Geometry: final body of the model. Coordinates: model frame, mm. A direction names the side the tool comes from. Coordinates: 2 decimals unless noted, no trailing zeros. Order: outer loops, then holes, each group sorted by start corner. A loop starts at its lowest first (then second) coordinate and runs counter-clockwise, first axis right, second up. Notation, with made-up numbers: (75.5, -27) - (94.5, -27) arc R23 ccw to (94.5, 7) - close; hole circle Ø2 at (70, 63.25). An arc over 180 degrees is marked (long way). Use a Markdown table: item, result. Add a question column.
Autodesk Inventor part; units mm, degrees
ref_plane "Work Plane1" through (0, 20, 0) normal (0, -1, 0) x (1, 0, 0)
ref_plane "YZ Plane" through (0, 0, 0) normal (1, 0, 0) x (0, 1, 0)
ref_plane "XZ Plane" through (0, 0, 0) normal (0, 1, 0) x (-1, 0, 0)
sketch "Sketch1" plane through (0, 0, 0) normal (0, 1, 0) x (-1, 0, 0)
  circle A0 centre (0, 0) radius 34.5
  dimension "d0" = 69
extrude "Extrusion1" add sketch "Sketch1" along normal blind 33.9
sketch "Sketch2" plane through (0, 33.9, 0) normal (0, 1, 0) x (1, 0, 0)
  circle A0 centre (0, 0) radius 34.5
  line L0 (-15, -15) -> (15, -15)
  line L1 (15, -15) -> (15, 15)
  line L2 (15, 15) -> (-15, 15)
  line L3 (-15, 15) -> (-15, -15)
  line L4 (-15, -15) -> (15, 15) construction
  line L5 (15, -15) -> (-15, 15) construction
  circle A1 centre (-15, 15) radius 1.5
  circle A2 centre (15, 15) radius 1.5
  circle A3 centre (-15, -15) radius 1.5
  circle A4 centre (15, -15) radius 1.5
  dimension "d3" = 30
  dimension "d4" = 30
  dimension "d5" = 3
  dimension "d6" = 3
  dimension "d7" = 3
  dimension "d8" = 3
hole "Hole1" at (-15, 33.9, 15) at (15, 33.9, 15) at (-15, 33.9, -15) at (15, 33.9, -15) direction (0, -1, 0) diameter 3 depth 10.4
sketch "Sketch3" plane through (0, 0, 0) normal (0, -1, 0) x (1, 0, 0)
  circle A0 centre (0, 0) radius 34.5
  circle A1 centre (0, 0) radius 6.35
  dimension "d16" = 12.7
extrude "Extrusion2" cut sketch "Sketch3" against normal blind 20 contours A1
ref_plane "Work Plane1" through (0, 20, 0) normal (0, -1, 0) x (1, 0, 0)
sketch "Sketch4" plane through (0, 20, 0) normal (0, -1, 0) x (1, 0, 0)
  circle A0 centre (0, 0) radius 6.35
  circle A1 centre (0, 0) radius 34.5
  circle A2 centre (0, 0) radius 34
  dimension "d20" = 68
extrude "Extrusion3" cut sketch "Sketch4" along normal mid plane 2 contours A1
sketch "Sketch5" plane through (0, 0, 0) normal (0, -1, 0) x (1, 0, 0)
  circle A0 centre (0, 0) radius 6.35
  circle A1 centre (0, 0) radius 34.5
  circle A2 centre (0, 0) radius 12.5
  line L0 (0, -1) -> (0, -12.5)
  circle A3 centre (0, -12.5) radius 2
  circle A4 centre (12.5, 0) radius 2
  circle A5 centre (0, 12.5) radius 2
  circle A6 centre (-12.5, 0) radius 2
  dimension "d23" = 25
  dimension "d24" = 4
  dimension "d27" = 360
hole "Hole2" at (0, 0, -12.5) at (12.5, 0, 0) at (0, 0, 12.5) at (-12.5, 0, 0) direction (0, 1, 0) diameter 3 depth 3.5
sketch "Sketch6" plane through (0, 0, 0) normal (0, -1, 0) x (1, 0, 0)
  line L0 (-63, 66) -> (64.0177, 66) construction
  line L1 (64.0177, 66) -> (64.0177, -63.3993) construction
  line L2 (64.0177, -63.3993) -> (-63, -63.3993) construction
  line L3 (-63, -63.3993) -> (-63, 66) construction
  point P0 (0, 0)
decal "Decal1"
properties part number "motor"
1) Section B-B (y = 28.5). Return loops of the section in (x, z).
2) Section A-A (z = 0). Return loops of the section in (x, y), then the cut area to 3 significant figures.
3) Draft query along Y for faces 4 (the face through (18.28, 19.99, 28.67)), 5 (the face through (0, 2, 14)), 6 (the face through (25.39, 19, -22.84)), 7 (the face through (15, 23.5, 15)). Return one class per face: pulls with the +Y half, pulls with the -Y half, needs draft (parallel to the pull), parting line crosses it, or undercut.
4) Section D-D (y = 7.5). Return loops of the section in (x, z).
5) Section C-C (x = 24.5). Return loops of the section in (y, z).
6) Pin query (flat end, axial travel): pin 1 (20.5 mm diameter, centred on x = -16, z = -2, fed in from -Y); pin 2 (2.5 mm diameter, centred on x = 12.5, z = 0, fed in from -Y); pin 3 (3 mm diameter, centred on x = -5.5, y = 9.5, fed in from +Z); pin 4 (12 mm diameter, centred on y = 24.5, z = 15, fed in from +X). Return the tip coordinate at first contact, or that it passes through.
7) Ray query, line 1 along Z through (x, y) = (0, 2); line 2 along X through (y, z) = (29, 15); line 3 along X through (y, z) = (0.8, -12.5). Return the intervals inside material, ascending.
8) Set-up query: faces 1 (the face through (14, 2, 0)), 2 (the face through (14.93, 28.63, 13.5)), 3 (the face through (0, 0, -7)). Return all of +Z, -Z, +X, -X, +Y, -Y with unobstructed straight access to the full face (end or side cutting, diameter ignored); none if empty.
Values follow:
| question | item | result |
|---|---|---|
| 1 | outline | circle Ø69 at (0, 0); hole circle Ø3 at (-15, -15); hole circle Ø3 at (-15, 15); hole circle Ø3 at (15, -15); hole circle Ø3 at (15, 15) |
| 2 | outline | (-34.5, 0) - (-14, 0) - (-14, 3.5) - (-11, 3.5) - (-11, 0) - (-6.35, 0) - (-6.35, 20) - (6.35, 20) - (6.35, 0) - (11, 0) - (11, 3.5) - (14, 3.5) - (14, 0) - (34.5, 0) - (34.5, 19) - (34, 19) - (34, 21) - (34.5, 21) - (34.5, 33.9) - (-34.5, 33.9) - (-34.5, 21) - (-34, 21) - (-34, 19) - (-34.5, 19) - close |
| 2 | area | 2,060 mm² |
| 3 | face 4 | undercut |
| 3 | face 5 | needs draft |
| 3 | face 6 | undercut |
| 3 | face 7 | pulls with the +Y half |
| 4 | outline | circle Ø69 at (0, 0); hole circle Ø12.7 at (0, 0) |
| 5 | outline | (0, -24.29) - (19, -24.29) - (19, -23.57) - (21, -23.57) - (21, -24.29) - (33.9, -24.29) - (33.9, 24.29) - (21, 24.29) - (21, 23.57) - (19, 23.57) - (19, 24.29) - (0, 24.29) - close |
| 6 | pin 1 | stops at y = 0 |
| 6 | pin 2 | stops at y = 3.5 |
| 6 | pin 3 | stops at z = 34.27 |
| 6 | pin 4 | stops at x = 33.31 |
| 7 | line 1 | z = -34.5 to -14, -11 to -6.35, 6.35 to 11, 14 to 34.5 |
| 7 | line 2 | x = -31.07 to -16.5, -13.5 to 13.5, 16.5 to 31.07 |
| 7 | line 3 | x = -32.16 to -1.5, 1.5 to 32.16 |
| 8 | face 1 | -Y |
| 8 | face 2 | +Y |
| 8 | face 3 | +Z, -Z, +X, -X, -Y |
